```python
from build123d import *

# Parameters (mm, degrees)
SKETCH1_R            = 6.35
BOSS_EXTRUDE2_DEPTH  = 101.6
SKETCH5_R            = 5.08
BOSS_EXTRUDE14_DEPTH = 10.16
SKETCH9_R            = 5.08
BOSS_EXTRUDE15_DEPTH = 10.16


with BuildPart() as part:
    # Sketch1 → Boss-Extrude2 (new body)
    with BuildSketch(Plane.XY):
        with Locations((-5.49342359, 5.704709113)):
            Circle(SKETCH1_R)
    extrude(amount=BOSS_EXTRUDE2_DEPTH)

    # Sketch5 → Boss-Extrude14 (add)
    with BuildSketch(Plane.XY.offset(101.6)):
        with Locations((-5.49342359, 5.704709113)):
            Circle(SKETCH5_R)
    extrude(amount=BOSS_EXTRUDE14_DEPTH)

    # Sketch9 → Boss-Extrude15 (add)
    with BuildSketch(Plane(origin=(0, 0, 0), x_dir=(-1, 0, 0), z_dir=(0, 0, -1))):
        with Locations((5.49342359, 5.704709113)):
            Circle(SKETCH9_R)
    extrude(amount=BOSS_EXTRUDE15_DEPTH)


solid = part.part
```
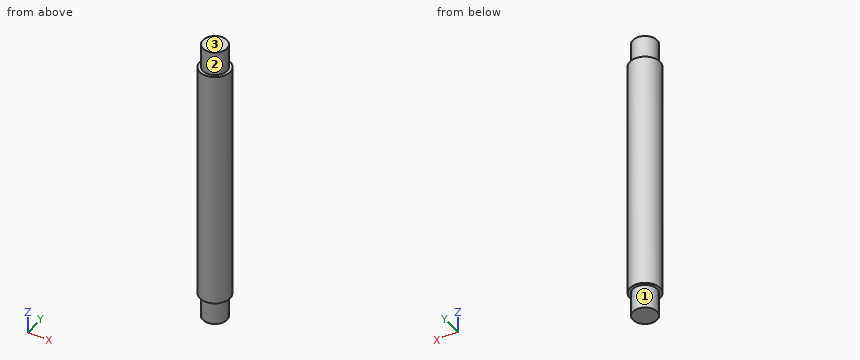
Verification items for the finished model (mm, model axes). Face numbers are marked on the shaded views. A direction names the side the tool comes from. Give positions to 0.01 mm unless a question says otherwise; leave off trailing zeros. Order: outer loops, then holes, each group sorted by start corner. A loop starts at its lowest first (then second) coordinate and runs counter-clockwise, first axis right, second up. Notation, with made-up numbers: M 50.25,-22 L 58.25,-22 A28 cw 58.25,15 Z; hole C -6,-30 d9. An arc over 180 degrees is marked long. Return JSON: item names as keys, results as strings. Group by question number.
1) Access from +Z, -Z, +X, -X, +Y, -Y to the whole of each face (thin tool, end or side, straight path). Record for the marked faces 1, 2 and 3.
2) Section check B-B on x = -3.25. Record the cut outline in (y, z).
3) Scan lines: line 1 (Z direction, x = -8.75, y = 10); line 2 (X direction, y = 4, z = 71.5); line 3 (Y direction, x = -2.75, z = 105). Record each from-to range of solid material in increasing order.
4) Section check C-C on z = 95.5. Record the cut outline in (x, y).
5) Section check A-A on y = 7. Record the cut outline in (x, z).
6) Go/stop test with flat-tipped pins: pin 1 Ø4 at (x, z) = (-4, 69.5) entering from -Y; pin 2 Ø3 at (y, z) = (2.5, 90.5) entering from +X; pin 3 Ø5 at (y, z) = (2.5, 37) entering from -X. Record where each tip stops, or that it passes through.
Answer block:
{
 "1": {"face 1": "-Z", "face 2": "+Z", "face 3": "+Z, +X, -X, +Y, -Y"},
 "2": {"outline": "M -0.24,0 L 1.15,0 L 1.15,-10.16 L 10.26,-10.16 L 10.26,0 L 11.65,0 L 11.65,101.6 L 10.26,101.6 L 10.26,111.76 L 1.15,111.76 L 1.15,101.6 L -0.24,101.6 Z"},
 "3": {"line 1": "z = 0 to 101.6", "line 2": "x = -11.61 to 0.62", "line 3": "y = 1.43 to 9.98"},
 "4": {"outline": "C -5.49,5.7 d12.7"},
 "5": {"outline": "M -11.71,0 L -10.41,0 L -10.41,-10.16 L -0.58,-10.16 L -0.58,0 L 0.72,0 L 0.72,101.6 L -0.58,101.6 L -0.58,111.76 L -10.41,111.76 L -10.41,101.6 L -11.71,101.6 Z"},
 "6": {"pin 1": "stops at y = -0.65", "pin 2": "stops at x = 0.62", "pin 3": "stops at x = -11.8"}
}
